from build123d import *

# Parameters (mm, degrees)
ESQUISSE1_W        = 45
ESQUISSE1_H        = 57
ESQUISSE1_R        = 1.6
BOSS_EXTRU_1_DEPTH = 1.6
ESQUISSE2_W        = 11.850194894
ESQUISSE2_H        = 3.329778143
ESQUISSE2_W_2      = 15.310163146
ESQUISSE2_H_2      = 36.439531762
ESQUISSE2_H_3      = 1.59771523
ESQUISSE2_W_3      = 9.88221832
ESQUISSE2_H_4      = 3.500525205
ESQUISSE2_W_4      = 7.70708484
ESQUISSE2_H_5      = 3.6703264
ESQUISSE2_H_6      = 3.670326401
ESQUISSE2_W_5      = 11.850194895
BOSS_EXTRU_2_DEPTH = 23.4


with BuildPart() as part:
    # Esquisse1 → Boss.-Extru.1 (new body)
    with BuildSketch(Plane.XY):
        Rectangle(ESQUISSE1_W, ESQUISSE1_H)
        with Locations(Location((13.5, 24.5, 0), (0, 0, 180))):
            Circle(ESQUISSE1_R, mode=Mode.SUBTRACT)
        with Locations((13.5, -24.5)):
            Circle(ESQUISSE1_R, mode=Mode.SUBTRACT)
        with Locations((-9.5, -24.5)):
            Circle(ESQUISSE1_R, mode=Mode.SUBTRACT)
    extrude(amount=BOSS_EXTRU_1_DEPTH)

    # Esquisse2 → Boss.-Extru.2 (add)
    with BuildSketch(Plane.XY.offset(1.6)):
        with Locations((14.82837193, 4.125238088)):
            Rectangle(ESQUISSE2_W, ESQUISSE2_H)
        Rectangle(ESQUISSE2_W_2, ESQUISSE2_H_2)
        with Locations((0, -20.508898976)):
            Rectangle(ESQUISSE2_W_2, ESQUISSE2_H_3)
        with Locations((14.82837193, 9.066341161)):
            Rectangle(ESQUISSE2_W, ESQUISSE2_H)
        with Locations((1.45328533, -24.82991901)):
            Rectangle(ESQUISSE2_W_3, ESQUISSE2_H_4)
        with Locations((16.899926957, -0.541039394)):
            Rectangle(ESQUISSE2_W_4, ESQUISSE2_H_5)
        with Locations((16.899926957, -5.483268114)):
            Rectangle(ESQUISSE2_W_4, ESQUISSE2_H_5)
        with Locations((16.899926957, -9.959457009)):
            Rectangle(ESQUISSE2_W_4, ESQUISSE2_H_5)
        with Locations((16.899926957, -14.89838332)):
            Rectangle(ESQUISSE2_W_4, ESQUISSE2_H_6)
        with Locations((-14.971381513, 24.411505641)):
            Rectangle(ESQUISSE2_W_5, ESQUISSE2_H)
        with Locations((-17.042936541, 14.467204765)):
            Rectangle(ESQUISSE2_W_4, ESQUISSE2_H_5)
        with Locations((-14.971381513, 19.461546453)):
            Rectangle(ESQUISSE2_W_5, ESQUISSE2_H)
        with Locations((-14.971381513, 9.066341161)):
            Rectangle(ESQUISSE2_W_5, ESQUISSE2_H)
        with Locations((-14.971381513, 4.116381974)):
            Rectangle(ESQUISSE2_W_5, ESQUISSE2_H)
        with Locations((-14.971381513, -0.370765265)):
            Rectangle(ESQUISSE2_W_5, ESQUISSE2_H)
        with Locations((-14.971381513, -5.320724453)):
            Rectangle(ESQUISSE2_W_5, ESQUISSE2_H)
        with Locations((-17.042936541, -10.31506614)):
            Rectangle(ESQUISSE2_W_4, ESQUISSE2_H_5)
        with Locations((-17.042936541, -15.126670853)):
            Rectangle(ESQUISSE2_W_4, ESQUISSE2_H_5)
    extrude(amount=BOSS_EXTRU_2_DEPTH)


solid = part.part
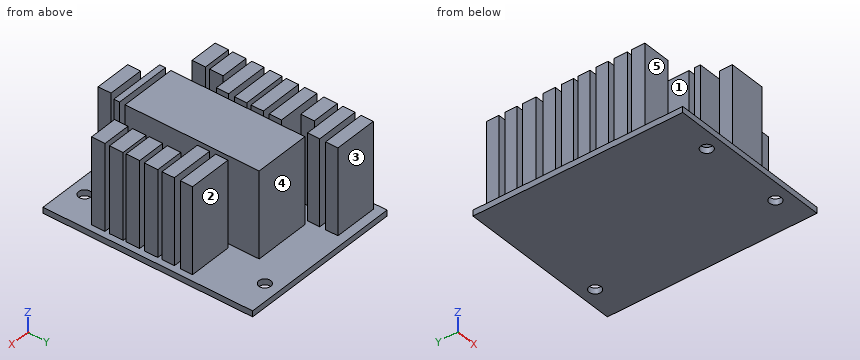
Can you work these out from the model? Positions are in its coordinate system, mm. Face numbers are marked on the shaded views. A direction names the side the tool comes from. Coordinates: 2 decimals unless noted, no trailing zeros. Order: outer loops, then holes, each group sorted by start corner. A loop starts at its lowest first (then second) coordinate and runs counter-clockwise, first axis right, second up. Notation, with made-up numbers: (21.25, 52.25) -> (67.25, 52.25) arc R16 cw to (67.25, 70.25) -> close; hole circle Ø10 at (60.25, 55). An arc over 180 degrees is marked (long way). Use one line per item in the form item = value.
Q1. Which directions (+Z, -Z, +X, -X, +Y, -Y) give clear straight access to the entire face, cutting with the end or side of a thin tool? Please do the marked faces 3, 4 and 5.
From the geometry:
face_3 = +Z, +X, -X, +Y
face_4 = +Z, +X, +Y
face_5 = +Z, -X, -Y
Q2. Imagine slicing it at C-C, the plane z = 6. Give the number of separate pieces and of enclosed holes in the cut face, then the cut area to 3 significant figures.
From the geometry:
separate_pieces = 18
enclosed_holes = 0
area = 1,130 mm²
Q3. Imagine slicing it at A-A, the plane y = 24.5. List the corners of the cut face in (x, z) for me.
From the geometry:
outline = (-22.5, 0) -> (11.9, 0) -> (11.9, 1.6) -> (-9.05, 1.6) -> (-9.05, 25) -> (-20.9, 25) -> (-20.9, 1.6) -> (-22.5, 1.6) -> close; (15.1, 0) -> (22.5, 0) -> (22.5, 1.6) -> (15.1, 1.6) -> close
Q4. Will these pins go through, and if not, where does the flat tip stop? P1, Ø4, axis at y = -6.5, z = 7, coming from the +X side; P2, Ø3, axis at y = -1.5, z = 17.5, coming from the -X side; P3, Ø4, axis at x = -17, z = 10.5, coming from the -Y side.
From the geometry:
P1 = 20.75
P2 = -20.9
P3 = -16.96
Q5. We'd pull the mould along X, two halves only. Please class the marked faces 1 and 2: released by +X, released by -X, zero draft, split by the parting line, or undercut.
From the geometry:
face_1 = undercut
face_2 = zero draft
Q6. I need wall thicknesses on L1, parallel to X at y = -10.5, z = 13.75; L2, parallel to X at y = -1.5, z = 4.5; L3, parallel to Y at x = 13.5, z = 1.1. Which ranges of each line are inside material? Lowest first, please.
From the geometry:
L1 = -20.9 to -13.19, -7.66 to 7.66, 13.05 to 20.75
L2 = -20.9 to -9.05, -7.66 to 7.66, 13.05 to 20.75
L3 = -28.5 to -26.1, -22.9 to 22.9, 26.1 to 28.5
Q7. Imagine slicing it at D-D, the plane x = 3.5. List the corners of the cut face in (y, z) for me, then the cut area to 3 significant figures.
From the geometry:
outline = (-28.5, 0) -> (28.5, 0) -> (28.5, 1.6) -> (18.22, 1.6) -> (18.22, 25) -> (-18.22, 25) -> (-18.22, 1.6) -> (-19.71, 1.6) -> (-19.71, 25) -> (-21.31, 25) -> (-21.31, 1.6) -> (-23.08, 1.6) -> (-23.08, 25) -> (-26.58, 25) -> (-26.58, 1.6) -> (-28.5, 1.6) -> close
area = 1,060 mm²
